```python
from build123d import *

# Parameters (mm, degrees)
BOSS_EXTRUDE1_DEPTH = 6.5


with BuildPart() as part:
    # Sketch1 → Boss-Extrude1 (new body, symmetric)
    with BuildSketch(Plane(origin=(0, 0, 0), x_dir=(1, 0, 0), z_dir=(0, 1, 0))):
        with BuildLine():
            Line((0, -242), (0, 242))
            Line((0, 242), (-46, 242))
            Line((-46, 242), (-46, 233.387339641))
            Line((-46, 233.387339641), (-372, 233.387339641))
            ThreePointArc((-372, 233.387339641), (-412.448780149, 221.907536408), (-440.836676218, 190.891136639))
            ThreePointArc((-440.836676218, 190.891136639), (-486, 0), (-440.836676218, -190.891136639))
            ThreePointArc((-440.836676218, -190.891136639), (-412.448780149, -221.907536408), (-372, -233.387339641))
            Line((-372, -233.387339641), (-46, -233.387339641))
            Line((-46, -233.387339641), (-46, -242))
            Line((-46, -242), (0, -242))
        make_face()
    extrude(amount=BOSS_EXTRUDE1_DEPTH, both=True)


solid = part.part
```
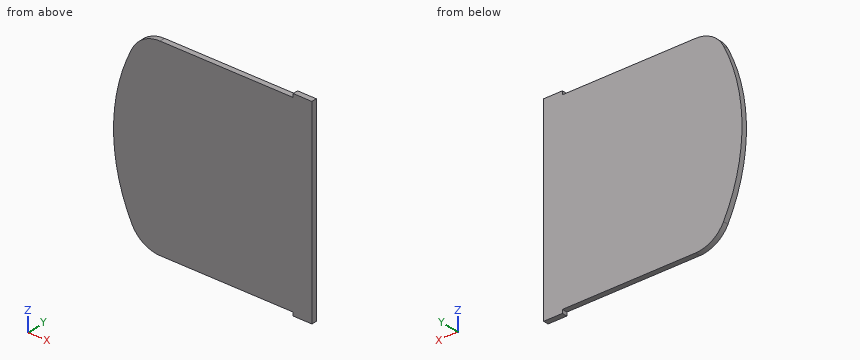
Can you work these out from the model? Positions are in its coordinate system, mm. Coordinates: 2 decimals unless noted, no trailing zeros. Order: outer loops, then holes, each group sorted by start corner. A loop starts at its lowest first (then second) coordinate and runs counter-clockwise, first axis right, second up.
1. If we section it at C-C (z = -93.5): Please give me the cut outline in (x, y).
2. If we section it at A-A (y = 2.25): Please give me the cut outline in (x, z).
3. I'm going to push flat-ended pins straight in: pin 1 (1.5 mm diameter, centred on x = -102, y = -3.5, fed in from -Z); pin 2 (7 mm diameter, centred on y = 3, z = 238.5, fed in from -X); pin 3 (3 mm diameter, centred on y = -3.5, z = -96, fed in from -X). Where does each tip first touch, or does it pass through?
4. If we section it at B-B (x = -210.5): Please give me the cut outline in (y, z).
5. I need wall thicknesses on line 1 (Z direction, x = -255, y = 1.25); line 2 (Z direction, x = -442, y = 6); line 3 (X direction, y = -4.25, z = 56.5). Which ranges of each line are inside material? Lowest first, please.
Entries:
1. outline: (-475.61, -6.5) - (0, -6.5) - (0, 6.5) - (-475.61, 6.5) - close
2. outline: (-440.84, -190.89) arc R77 ccw to (-372, -233.39) - (-46, -233.39) - (-46, -242) - (0, -242) - (0, 242) - (-46, 242) - (-46, 233.39) - (-372, 233.39) arc R77 ccw to (-440.84, 190.89) arc R426 ccw to start
3. pin 1: stops at z = -233.39
3. pin 2: stops at x = -46
3. pin 3: stops at x = -475.39
4. outline: (-6.5, -233.39) - (6.5, -233.39) - (6.5, 233.39) - (-6.5, 233.39) - close
5. line 1: z = -233.39 to 233.39
5. line 2: z = -188.55 to 188.55
5. line 3: x = -482.24 to 0
